from build123d import *

# Parameters (mm, degrees)
SZKIC1_W                        = 28
SZKIC1_H                        = 16
DODANIE_WYCI_GNI_CIE1_DEPTH     = 10
WYTNIJ_WYCI_GNI_CIE1_REACH      = 12
SZKIC2_R                        = 1.7
ZAOKR_GLENIE1_R                 = 3
WYTNIJ_WYCI_GNI_CIE2_DEPTH      = 4
WYTNIJ_WYCI_GNI_CIE2_DEPTH_BACK = 4
WYTNIJ_WYCI_GNI_CIE3_DEPTH      = 3
WYTNIJ_WYCI_GNI_CIE4_REACH      = 18
SZKIC5_W                        = 2
SZKIC5_H                        = 4.5
SZKIC5_W_2                      = 3
SZKIC6_R                        = 2
WYTNIJ_WYCI_GNI_CIE5_DEPTH      = 0.5
WYTNIJ_WYCI_GNI_CIE6_REACH      = 11.5
SZKIC7_R                        = 1
WYTNIJ_WYCI_GNI_CIE7_REACH      = 30
SZKIC8_W                        = 5
SZKIC8_H                        = 1
WYTNIJ_WYCI_GNI_CIE8_REACH      = 18
SZKIC9_W                        = 1
SZKIC9_H                        = 5


with BuildPart() as part:
    # Szkic1 → Dodanie-wyciągnięcie1 (new body)
    with BuildSketch(Plane.XY):
        Rectangle(SZKIC1_W, SZKIC1_H)
    extrude(amount=DODANIE_WYCI_GNI_CIE1_DEPTH)

    # Szkic2 → Wytnij-wyciągnięcie1 (cut, up to next)
    with BuildSketch(Plane.XY.offset(10), mode=Mode.PRIVATE) as wytnij_wyci_gni_cie1_sk1:
        with Locations((-11, 5)):
            Circle(SZKIC2_R)
    wytnij_wyci_gni_cie1_tool1 = extrude(wytnij_wyci_gni_cie1_sk1.sketch, amount=-WYTNIJ_WYCI_GNI_CIE1_REACH, mode=Mode.PRIVATE) & part.part
    add(wytnij_wyci_gni_cie1_tool1.solids().sort_by_distance((-11, 5, 10))[0], mode=Mode.SUBTRACT)
    # Szkic2 → Wytnij-wyciągnięcie1 (cut, up to next)
    with BuildSketch(Plane.XY.offset(10), mode=Mode.PRIVATE) as wytnij_wyci_gni_cie1_sk2:
        with Locations((11, -5)):
            Circle(SZKIC2_R)
    wytnij_wyci_gni_cie1_tool2 = extrude(wytnij_wyci_gni_cie1_sk2.sketch, amount=-WYTNIJ_WYCI_GNI_CIE1_REACH, mode=Mode.PRIVATE) & part.part
    add(wytnij_wyci_gni_cie1_tool2.solids().sort_by_distance((11, -5, 10))[0], mode=Mode.SUBTRACT)

    # Zaokrąglenie1
    zaokr_glenie1_edges = [part.edges().sort_by_distance(p)[0] for p in [
        (14, -8, 5),
        (-14, -8, 5),
        (-14, 8, 5),
        (14, 8, 5),
    ]]
    fillet(zaokr_glenie1_edges, radius=ZAOKR_GLENIE1_R)

    # Szkic3 → Wytnij-wyciągnięcie2 (cut, two sides)
    with BuildSketch(Plane.XY.offset(5)) as wytnij_wyci_gni_cie2_sk:
        with BuildLine():
            Line((11, 7), (-7.3, 7))
            ThreePointArc((-7.3, 7), (-8.007106781, 6.707106781), (-8.3, 6))
            Line((-8.3, 6), (-8.3, 5))
            ThreePointArc((-8.3, 5), (-9.090811691, 3.090811691), (-11, 2.3))
            Line((-11, 2.3), (-12, 2.3))
            ThreePointArc((-12, 2.3), (-12.707106781, 2.007106781), (-13, 1.3))
            Line((-13, 1.3), (-13, -5))
            ThreePointArc((-13, -5), (-12.414213562, -6.414213562), (-11, -7))
            Line((-11, -7), (7.3, -7))
            ThreePointArc((7.3, -7), (8.007106781, -6.707106781), (8.3, -6))
            Line((8.3, -6), (8.3, -5))
            ThreePointArc((8.3, -5), (9.090811691, -3.090811691), (11, -2.3))
            Line((11, -2.3), (12, -2.3))
            ThreePointArc((12, -2.3), (12.707106781, -2.007106781), (13, -1.3))
            Line((13, -1.3), (13, 5))
            ThreePointArc((13, 5), (12.414213562, 6.414213562), (11, 7))
        make_face()
    extrude(amount=WYTNIJ_WYCI_GNI_CIE2_DEPTH, mode=Mode.SUBTRACT)
    extrude(wytnij_wyci_gni_cie2_sk.sketch, amount=-WYTNIJ_WYCI_GNI_CIE2_DEPTH_BACK, mode=Mode.SUBTRACT)

    # Szkic4 → Wytnij-wyciągnięcie3 (cut)
    with BuildSketch(Plane(origin=(0, 0, 0), x_dir=(-1, 0, 0), z_dir=(0, 0, -1))):
        with BuildLine():
            Line((-11, 8), (8.3, 8))
            Line((8.3, 8), (8.3, 5))
            ThreePointArc((8.3, 5), (9.090811691, 3.090811691), (11, 2.3))
            Line((11, 2.3), (14, 2.3))
            Line((14, 2.3), (14, -5))
            ThreePointArc((14, -5), (13.121320344, -7.121320344), (11, -8))
            Line((11, -8), (-8.3, -8))
            Line((-8.3, -8), (-8.3, -5))
            ThreePointArc((-8.3, -5), (-9.090811691, -3.090811691), (-11, -2.3))
            Line((-11, -2.3), (-14, -2.3))
            Line((-14, -2.3), (-14, 5))
            ThreePointArc((-14, 5), (-13.121320344, 7.121320344), (-11, 8))
        make_face()
    extrude(amount=-WYTNIJ_WYCI_GNI_CIE3_DEPTH, mode=Mode.SUBTRACT)

    # Szkic5 → Wytnij-wyciągnięcie4 (cut, up to next)
    with BuildSketch(Plane(origin=(0, 8, 0), x_dir=(1, 0, 0), z_dir=(0, 1, 0)), mode=Mode.PRIVATE) as wytnij_wyci_gni_cie4_sk1:
        with Locations((3, -5.25)):
            Rectangle(SZKIC5_W, SZKIC5_H)
    wytnij_wyci_gni_cie4_tool1 = extrude(wytnij_wyci_gni_cie4_sk1.sketch, amount=-WYTNIJ_WYCI_GNI_CIE4_REACH, mode=Mode.PRIVATE) & part.part
    add(wytnij_wyci_gni_cie4_tool1.solids().sort_by_distance((3, 8, 5.25))[0], mode=Mode.SUBTRACT)
    # Szkic5 → Wytnij-wyciągnięcie4 (cut, up to next)
    with BuildSketch(Plane(origin=(0, 8, 0), x_dir=(1, 0, 0), z_dir=(0, 1, 0)), mode=Mode.PRIVATE) as wytnij_wyci_gni_cie4_sk2:
        with Locations((9.2, -5.25)):
            Rectangle(SZKIC5_W_2, SZKIC5_H)
    wytnij_wyci_gni_cie4_tool2 = extrude(wytnij_wyci_gni_cie4_sk2.sketch, amount=-WYTNIJ_WYCI_GNI_CIE4_REACH, mode=Mode.PRIVATE) & part.part
    add(wytnij_wyci_gni_cie4_tool2.solids().sort_by_distance((9.2, 8, 5.25))[0], mode=Mode.SUBTRACT)
    # Szkic5 → Wytnij-wyciągnięcie4 (cut, up to next)
    with BuildSketch(Plane(origin=(0, 8, 0), x_dir=(1, 0, 0), z_dir=(0, 1, 0)), mode=Mode.PRIVATE) as wytnij_wyci_gni_cie4_sk3:
        with Locations((-2.5, -5.25)):
            Rectangle(SZKIC5_W, SZKIC5_H)
    wytnij_wyci_gni_cie4_tool3 = extrude(wytnij_wyci_gni_cie4_sk3.sketch, amount=-WYTNIJ_WYCI_GNI_CIE4_REACH, mode=Mode.PRIVATE) & part.part
    add(wytnij_wyci_gni_cie4_tool3.solids().sort_by_distance((-2.5, 8, 5.25))[0], mode=Mode.SUBTRACT)

    # Szkic6 → Wytnij-wyciągnięcie5 (cut)
    with BuildSketch(Plane.XY.offset(10)):
        with Locations((0.5, 5.5)):
            Circle(SZKIC6_R)
    extrude(amount=-WYTNIJ_WYCI_GNI_CIE5_DEPTH, mode=Mode.SUBTRACT)

    # Szkic7 → Wytnij-wyciągnięcie6 (cut, up to next)
    with BuildSketch(Plane.XY.offset(9.5), mode=Mode.PRIVATE) as wytnij_wyci_gni_cie6_sk1:
        with Locations((0.5, 5.5)):
            Circle(SZKIC7_R)
    wytnij_wyci_gni_cie6_tool1 = extrude(wytnij_wyci_gni_cie6_sk1.sketch, amount=-WYTNIJ_WYCI_GNI_CIE6_REACH, mode=Mode.PRIVATE) & part.part
    add(wytnij_wyci_gni_cie6_tool1.solids().sort_by_distance((0.5, 5.5, 9.5))[0], mode=Mode.SUBTRACT)

    # Szkic8 → Wytnij-wyciągnięcie7 (cut, up to next)
    with BuildSketch(Plane.ZY.offset(14), mode=Mode.PRIVATE) as wytnij_wyci_gni_cie7_sk1:
        with Locations((5.5, 1.6)):
            Rectangle(SZKIC8_W, SZKIC8_H)
    wytnij_wyci_gni_cie7_tool1 = extrude(wytnij_wyci_gni_cie7_sk1.sketch, amount=-WYTNIJ_WYCI_GNI_CIE7_REACH, mode=Mode.PRIVATE) & part.part
    add(wytnij_wyci_gni_cie7_tool1.solids().sort_by_distance((-14, 1.6, 5.5))[0], mode=Mode.SUBTRACT)
    # Szkic8 → Wytnij-wyciągnięcie7 (cut, up to next)
    with BuildSketch(Plane.ZY.offset(14), mode=Mode.PRIVATE) as wytnij_wyci_gni_cie7_sk2:
        with Locations((5.5, -3.8)):
            Rectangle(SZKIC8_W, SZKIC8_H)
    wytnij_wyci_gni_cie7_tool2 = extrude(wytnij_wyci_gni_cie7_sk2.sketch, amount=-WYTNIJ_WYCI_GNI_CIE7_REACH, mode=Mode.PRIVATE) & part.part
    add(wytnij_wyci_gni_cie7_tool2.solids().sort_by_distance((-14, -3.8, 5.5))[0], mode=Mode.SUBTRACT)

    # Szkic9 → Wytnij-wyciągnięcie8 (cut, up to next)
    with BuildSketch(Plane.XZ.offset(8), mode=Mode.PRIVATE) as wytnij_wyci_gni_cie8_sk1:
        with Locations((-2, 5.5)):
            Rectangle(SZKIC9_W, SZKIC9_H)
    wytnij_wyci_gni_cie8_tool1 = extrude(wytnij_wyci_gni_cie8_sk1.sketch, amount=-WYTNIJ_WYCI_GNI_CIE8_REACH, mode=Mode.PRIVATE) & part.part
    add(wytnij_wyci_gni_cie8_tool1.solids().sort_by_distance((-2, -8, 5.5))[0], mode=Mode.SUBTRACT)


solid = part.part
Input: part model. Units: mm. Frame: model coordinates. A direction names the side the tool comes from. Round coordinates to 2 decimals unless told otherwise and drop trailing zeros. Loops run counter-clockwise (first coordinate to the right, second up) from the corner with the lowest first, then second, coordinate; pieces in that order, holes last. Notation, with made-up numbers: (79.25, 12.25) -> (83.25, 12.25) arc R17 ccw to (83.25, 30.25) -> close; hole circle Ø7 at (-39, 32). An arc over 180 degrees is marked (long way). Answer as a JSON object with one key per item and string values. Group by question number.
1) Reachability of faces 1 (the flat face through (-5.9, 7.5, 3)), 2 (the flat face through (-8.3, 5.85, 3.44)), 3 (the flat face through (13.3, 3.3, 3)), 4 (the flat face through (7.7, 7.5, 5.3)), 5 (the cylindrical face through (12.57, -5.65, 5.07)) from +Z, -Z, +X, -X, +Y, -Y: full face, straight path, thin tool, end or side. Return the list, or none.
2) Section query B-B on z = 6.75. State how many separate pieces and enclosed holes the cut face has, plus the area to 3 significant figures.
3) Section query C-C on x = 6.5. Output: boundary loops of the cut face in (y, z).
4) Draft query along Y for faces 6 (the flat face through (-13.5, 1.6, 8)), 7 (the cylindrical face through (13.1, -7.14, 5.07)), 8 (the flat face through (-9.1, -7.4, 3)). Return one class per face: +Y half, -Y half, draft (parallel to the pull), parting line (faces both ways), or undercut.
5) Section query D-D on y = 5.5. Output: boundary loops of the cut face in (x, z).
6) Section query A-A on z = 1. Output: boundary loops of the cut face in (x, y).
7) Ray query, L1, parallel to Y at x = 11, z = 3.5; L2, parallel to Y at x = -11, z = 5.25; L3, parallel to X at y = -5.75, z = 4. Return the intervals inside material, ascending.
8) Pin query (flat end, axial travel): pin 1 (1.2 mm diameter, centred on x = 1, y = 5.5, fed in from +Z); pin 2 (3 mm diameter, centred on x = -2, y = -1, fed in from -Z); pin 3 (1.5 mm diameter, centred on x = -13.5, z = 4.5, fed in from -Y). Return the tip coordinate at first contact, or that it passes through.
Reply:
{
 "1": {"face 1": "-Z, +X, +Y, -Y", "face 2": "-Z", "face 3": "-Z, +X, +Y", "face 4": "-Z, +Y", "face 5": "+Z, -Z"},
 "2": {"separate pieces": "6", "enclosed holes": "2", "area": "91.6 mm2"},
 "3": {"outline": "(-8, 3) -> (-7, 3) -> (-7, 9) -> (7, 9) -> (7, 3) -> (8, 3) -> (8, 10) -> (-8, 10) -> close"},
 "4": {"face 6": "undercut", "face 7": "-Y half", "face 8": "draft"},
 "5": {"outline": "(-13.96, 0) -> (-12.62, 0) -> (-12.62, 10) -> (-13.96, 10) -> close; (-9.38, 0) -> (-8.3, 0) -> (-8.3, 9) -> (-0.5, 9) -> (-0.5, 9.5) -> (-1.5, 9.5) -> (-1.5, 10) -> (-9.38, 10) -> close; (1.5, 9) -> (12.94, 9) -> (12.94, 3) -> (13.96, 3) -> (13.96, 10) -> (2.5, 10) -> (2.5, 9.5) -> (1.5, 9.5) -> close"},
 "6": {"outline": "(-14, 2.3) -> (-11, 2.3) arc R2.7 ccw to (-8.3, 5) -> (-8.3, 8) -> (-11, 8) arc R3 ccw to (-14, 5) -> close; (8.3, -8) -> (11, -8) arc R3 ccw to (14, -5) -> (14, -2.3) -> (11, -2.3) arc R2.7 ccw to (8.3, -5) -> close; hole circle Ø3.4 at (-11, 5); hole circle Ø3.4 at (11, -5)"},
 "7": {"L1": "y = -8 to -6.7, -3.3 to -2.3, 7 to 8", "L2": "y = -8 to -7, 2.3 to 3.3, 6.7 to 8", "L3": "x = -13.9 to -12.85, 8.3 to 9.47, 12.53 to 13.9"},
 "8": {"pin 1": "stops at z = 9.5", "pin 2": "stops at z = 9", "pin 3": "stops at y = -7.44"}
}
